Check sheet for the modelled part. Datum: model origin and axes. Units: mm. A direction names the side the tool comes from. Give positions to 0.01 mm unless a question says otherwise; leave off trailing zeros. Loops run counter-clockwise (first coordinate to the right, second up) from the corner with the lowest first, then second, coordinate; pieces in that order, holes last. Notation, with made-up numbers: (4.25, -28.5) -> (33.25, -28.5) arc R21 ccw to (33.25, -16.5) -> close; hole circle Ø4 at (-3, 40.5). An arc over 180 degrees is marked (long way). Write each question's results on one line, items separated by ' | '. Start each with the question number.
1. Cross-section at B-B on z = 19.5. Record the boundary of the cut face in (x, y), and give its area (3 significant figures).
2. Mould release check, pull along Z, two halves, no side actions. Record for faces 1 (the face through (-22, 2.5, -8.5)), 2 (the face through (-10.54, 2.54, -7.56)), 3 (the face through (-22, 17, 16)), 4 (the face through (-23, 20, 19)): +Z half, -Z half, draft (parallel to the pull), parting line (faces both ways), or undercut.
3. Material ranges on L1, parallel to X at y = 3.5, z = -10; L2, parallel to Z at x = -20, y = 1.8; L3, parallel to Y at x = -26.5, z = -14, recorded low to high. Write a range as from..to.
4. Cross-section at D-D on z = -10. Record the boundary of the cut face in (x, y), and give its area (3 significant figures).
5. Gauge pin test, flat ends, axial feed: pin 1 Ø4.5 at (x, y) = (-33, 16.5) entering from -Z; pin 2 Ø11 at (x, z) = (-29.5, 3.5) entering from +Y; pin 3 Ø4 at (y, z) = (3.5, -5.5) entering from -X. Record the tip position at first contact, or that the pin passes through.
6. Tool access check on faces 5 (the face through (-23, 18, 10)), 6 (the face through (-30, 2, -10)), 7 (the face through (-23, 14, 20)). Record the directions out of +Z, -Z, +X, -X, +Y, -Y that give a thin tool (end or side, any length) a straight path to the whole face; none if there is none.
7. Cross-section at A-A on x = -20. Record the boundary of the cut face in (y, z), and give its area (3 significant figures).
8. Cross-section at C-C on y = 3. Record the boundary of the cut face in (x, z), and give its area (3 significant figures).
Autodesk Inventor part; units mm, degrees
ref_plane "YZ Plane" through (0, 0, 0) normal (1, 0, 0) x (0, 1, 0)
ref_plane "XZ Plane" through (0, 0, 0) normal (0, 1, 0) x (-1, 0, 0)
ref_plane "XY Plane" through (0, 0, 0) normal (0, 0, 1) x (1, 0, 0)
sketch "Esboço1" plane through (0, 0, 0) normal (0, 1, 0) x (-1, 0, 0)
  line L0 (0, 0) -> (0, -20)
  line L1 (0, -20) -> (30, -20)
  line L2 (30, -20) -> (30, 0)
  line L3 (30, 0) -> (0, 0)
  circle A0 centre (15, -10) radius 2.5
  dimension "d0" = 20
  dimension "d1" = 30
  dimension "d2" = 5
extrude "Extrusão1" add sketch "Esboço1" along normal blind 5
sketch "Esboço2" plane through (0, 0, 0) normal (0, -1, 0) x (1, 0, 0)
  line L0 (0, 0) -> (0, 23)
  line L1 (0, 23) -> (-45, 23)
  line L2 (-45, 23) -> (-45, 0)
  line L3 (-45, 0) -> (0, 0)
  dimension "d5" = 23
  dimension "d6" = 45
extrude "Extrusão2" add sketch "Esboço2" against normal blind 14
sketch "Esboço3" plane through (0, 14, 0) normal (0, 1, 0) x (1, 0, 0)
  line L0 (0, -23) -> (0, 20)
  line L1 (0, -23) -> (0, -16)
  line L2 (0, -16) -> (-45, -16)
  line L3 (-45, 0) -> (-45, -23)
  line L4 (-45, -16) -> (-45, -10)
  line L5 (-45, -10) -> (0, -10)
  line L6 (0, -10) -> (0, -16)
  point P0 (0, 0)
  dimension "d9" = 7
  dimension "d10" = 6
extrude "Extrusão3" add sketch "Esboço3" along normal blind 6
sketch "Esboço4" plane through (0, 20, 0) normal (0, 1, 0) x (1, 0, 0)
  line L0 (-45, -10) -> (0, -10)
  line L1 (-45, -23) -> (-45, 0)
  line L2 (-45, -10) -> (-45, -23)
  line L3 (-45, -23) -> (0, -23)
  line L4 (-45, -23) -> (0, -23)
  line L5 (0, -16) -> (0, -10)
  line L6 (0, -23) -> (0, -10)
  line L7 (0, -10) -> (-45, -10)
  point P0 (0, 0)
extrude "Extrusão4" add sketch "Esboço4" along normal blind 3
sketch "Esboço5" plane through (-45, 0, 0) normal (-1, 0, 0) x (0, 0, 1)
  line L0 (10, 14) -> (12.7, 14)
  line L1 (12.7, 14) -> (12.7, 9.5)
  line L2 (12.7, 9.5) -> (10, 9.5)
  line L3 (10, 14) -> (10, 23)
  line L4 (10, 9.5) -> (10, 14)
  point P0 (0, 0)
  dimension "d15" = 2.7
  dimension "d16" = 4.5
extrude "Extrusão5" add sketch "Esboço5" along normal blind 10
offset faces "Tamanho1" outward -10 faces at (-55, 12.5, 10.9)
sketch "Esboço6" plane through (0, 5, 0) normal (0, 1, 0) x (1, 0, 0)
  line L0 (0, -23) -> (0, 20)
  line L1 (0, 20) -> (-15, 20)
  line L2 (0, 20) -> (-30, 20)
  line L3 (-15, 20) -> (-15, 10)
  circle A0 centre (-15, 10) radius 2.5
  point P0 (0, 0)
  dimension "d20" = 10
extrude "Extrusão6" add sketch "Esboço6" against normal blind 5
sketch "Esboço7" plane through (0, 5, 0) normal (0, 1, 0) x (1, 0, 0)
  line L0 (0, 20) -> (-30, 20)
  line L1 (0, 20) -> (-10, 20)
  line L2 (-10, 20) -> (-20, 20)
  line L3 (-20, 20) -> (-20, 10)
  line L4 (-10, 20) -> (-10, 10)
  circle A0 centre (-10, 10) radius 2.5
  circle A1 centre (-20, 10) radius 2.5
  point P0 (0, 0)
  dimension "d23" = 10
  dimension "d24" = 10
  dimension "d25" = 10
  dimension "d26" = 5
extrude "Extrusão7" cut sketch "Esboço7" against normal blind 5
properties part number "suporte p trilho"
Geometry says:
1) outline: (-45, 0) -> (0, 0) -> (0, 14) -> (-45, 14) -> close; (-45, 20) -> (0, 20) -> (0, 23) -> (-45, 23) -> close | area: 765 mm^2
2) face 1: undercut | face 2: undercut | face 3: +Z half | face 4: draft
3) L1: -30..-22.5, -17.5..-12.5, -7.5..0 | L2: -20..-12.5, -7.5..23 | L3: 0..5
4) outline: (-30, 0) -> (-22.5, 0) -> (-22.5, 5) -> (-30, 5) -> close; (-17.5, 0) -> (-12.5, 0) -> (-12.5, 5) -> (-17.5, 5) -> close; (-7.5, 0) -> (0, 0) -> (0, 5) -> (-7.5, 5) -> close | area: 100 mm^2
5) pin 1: z = 10 | pin 2: y = 14 | pin 3: x = -30
6) face 5: -Z, +X, -X, +Y | face 6: -Z, -X, +Y, -Y | face 7: +Z, +X, -X
7) outline: (0, -20) -> (5, -20) -> (5, -12.5) -> (0, -12.5) -> close; (0, -7.5) -> (5, -7.5) -> (5, 0) -> (14, 0) -> (14, 10) -> (23, 10) -> (23, 23) -> (20, 23) -> (20, 16) -> (14, 16) -> (14, 23) -> (0, 23) -> close | area: 472 mm^2
8) outline: (-45, 0) -> (-30, 0) -> (-30, -20) -> (0, -20) -> (0, 23) -> (-45, 23) -> close; hole circle Ø5 at (-20, -10); hole circle Ø5 at (-10, -10) | area: 1,600 mm^2
